Autodesk Inventor part; units mm, degrees
ref_plane "YZ Plane" through (0, 0, 0) normal (1, 0, 0) x (0, 1, 0)
ref_plane "XZ Plane" through (0, 0, 0) normal (0, 1, 0) x (-1, 0, 0)
ref_plane "XY Plane" through (0, 0, 0) normal (0, 0, 1) x (1, 0, 0)
sketch "Эскиз1" plane through (0, 0, 0) normal (0, 0, 1) x (1, 0, 0)
  circle A0 centre (0, 0) radius 2.1
  line L0 (-31.5, -5) -> (31.5, -5)
  line L1 (31.5, -5) -> (31.5, 5)
  line L2 (31.5, 5) -> (-31.5, 5)
  line L3 (-31.5, 5) -> (-31.5, -5)
  line L4 (-31.5, -5) -> (31.5, 5) construction
  line L5 (31.5, -5) -> (-31.5, 5) construction
  line L6 (-7, 5) -> (-7, -5)
  dimension "d0" = 4.2
  dimension "d1" = 63
  dimension "d2" = 10
  dimension "d3" = 7
extrude "Выдавливание1" add sketch "Эскиз1" along normal blind 3.2 contours L6 L2 L1 L0
sketch "Эскиз2" plane through (0, 0, 0) normal (0, 0, -1) x (-1, 0, 0)
  line L0 (-31.5, 5) -> (7, 5)
  line L1 (7, -5) -> (-31.5, -5)
  line L2 (-31.5, 5) -> (-28.3, 5)
  line L3 (-28.3, 5) -> (-28.3, -5)
  line L4 (-28.3, -5) -> (-31.5, -5)
  line L5 (-31.5, -5) -> (-31.5, 5)
  point P0 (0, 0)
  point P1 (-28.3, 5)
  dimension "d6" = 3.2
extrude "Выдавливание2" add sketch "Эскиз2" along normal blind 13
fillet "Сопряжение1" radius 3 1 edges at (28.3, 0, 0)
sketch "Эскиз3" plane through (28.3, -5, -13) normal (-1, 0, 0) x (0, 0, 1)
  line L0 (0, 0) -> (0, 10)
  line L1 (0, 5) -> (10, 5)
  line L2 (10, 10) -> (10, 0)
  circle A0 centre (5, 5) radius 2.1
  point P0 (13, 5)
  dimension "d10" = 4.2
extrude "Выдавливание3" cut sketch "Эскиз3" against normal blind 13
properties part number "мертвое колесо крепл 2 25-26"
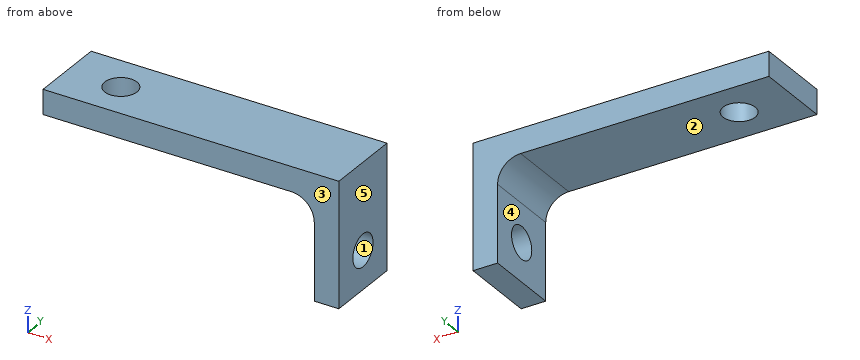
Design review of the part built by this model. Coordinates are the model's own, in mm. Face numbers are marked on the shaded views. A direction names the side the tool comes from. Coordinates: 2 decimals unless noted, no trailing zeros. Loops run counter-clockwise (first coordinate to the right, second up) from the corner with the lowest first, then second, coordinate; pieces in that order, holes last. Notation, with made-up numbers: (86, 29.25) -> (90, 29.25) arc R14 cw to (90, 37.25) -> close; hole circle Ø10 at (46, 84). An arc over 180 degrees is marked (long way). Use a Markdown table: item, result. Add a question column.
Item 1: Machinability: for the marked faces 4 and 5, which of the approach directions +Z, -Z, +X, -X, +Y, -Y give a long, thin tool a straight path to every point of the face, cutting with its end or side? Answer none if there is none.
Item 2: The part is to be moulded in two halves that separate along Y. For the marked faces 1, 2 and 3, say which applies: +Y half, -Y half, draft (parallel to the pull), parting line (faces both ways), or undercut.
Item 3: We need section C-C, the plane x = 0. Write out the cut boundary in (y, z).
Item 4: Clearance check with flat-ended pins moving along their axes: P1, Ø2.5, axis at x = 0, y = 0, coming from the -Z side; P2, Ø5, axis at y = -1, z = -7, coming from the -X side. State where each tip first meets the part, or that it passes through.
Item 5: Wall thickness on L1, parallel to Y at x = 30.1, z = -8; L2, parallel to Z at x = 30.65, y = 0; L3, parallel to Z at x = 25, y = -1.25: over which ranges is each line inside the solid? List them lowest first. Write a range as from..to.
Item 6: We need section B-B, the plane z = -8. Write out the cut boundary in (x, y).
Item 7: We need section A-A, the plane y = 0. Write out the cut boundary in (x, z).
Item 8: We need section D-D, the plane y = -3.25. Write out the cut boundary in (x, z).
Numbers:
| question | item | result |
|---|---|---|
| 1 | face 4 | -Z, -X, +Y, -Y |
| 1 | face 5 | +Z, -Z, +X, +Y, -Y |
| 2 | face 1 | undercut |
| 2 | face 2 | draft |
| 2 | face 3 | -Y half |
| 3 | outline | (-5, 0) -> (-2.1, 0) -> (-2.1, 3.2) -> (-5, 3.2) -> close; (2.1, 0) -> (5, 0) -> (5, 3.2) -> (2.1, 3.2) -> close |
| 4 | P1 | passes through |
| 4 | P2 | stops at x = 28.3 |
| 5 | L1 | y = -5..-2.1, 2.1..5 |
| 5 | L2 | z = -13..-10.1, -5.9..3.2 |
| 5 | L3 | z = 0..3.2 |
| 6 | outline | (28.3, -5) -> (31.5, -5) -> (31.5, -2.1) -> (28.3, -2.1) -> close; (28.3, 2.1) -> (31.5, 2.1) -> (31.5, 5) -> (28.3, 5) -> close |
| 7 | outline | (-7, 0) -> (-2.1, 0) -> (-2.1, 3.2) -> (-7, 3.2) -> close; (2.1, 0) -> (25.3, 0) arc R3 cw to (28.3, -3) -> (28.3, -5.9) -> (31.5, -5.9) -> (31.5, 3.2) -> (2.1, 3.2) -> close; (28.3, -13) -> (31.5, -13) -> (31.5, -10.1) -> (28.3, -10.1) -> close |
| 8 | outline | (-7, 0) -> (25.3, 0) arc R3 cw to (28.3, -3) -> (28.3, -13) -> (31.5, -13) -> (31.5, 3.2) -> (-7, 3.2) -> close |
